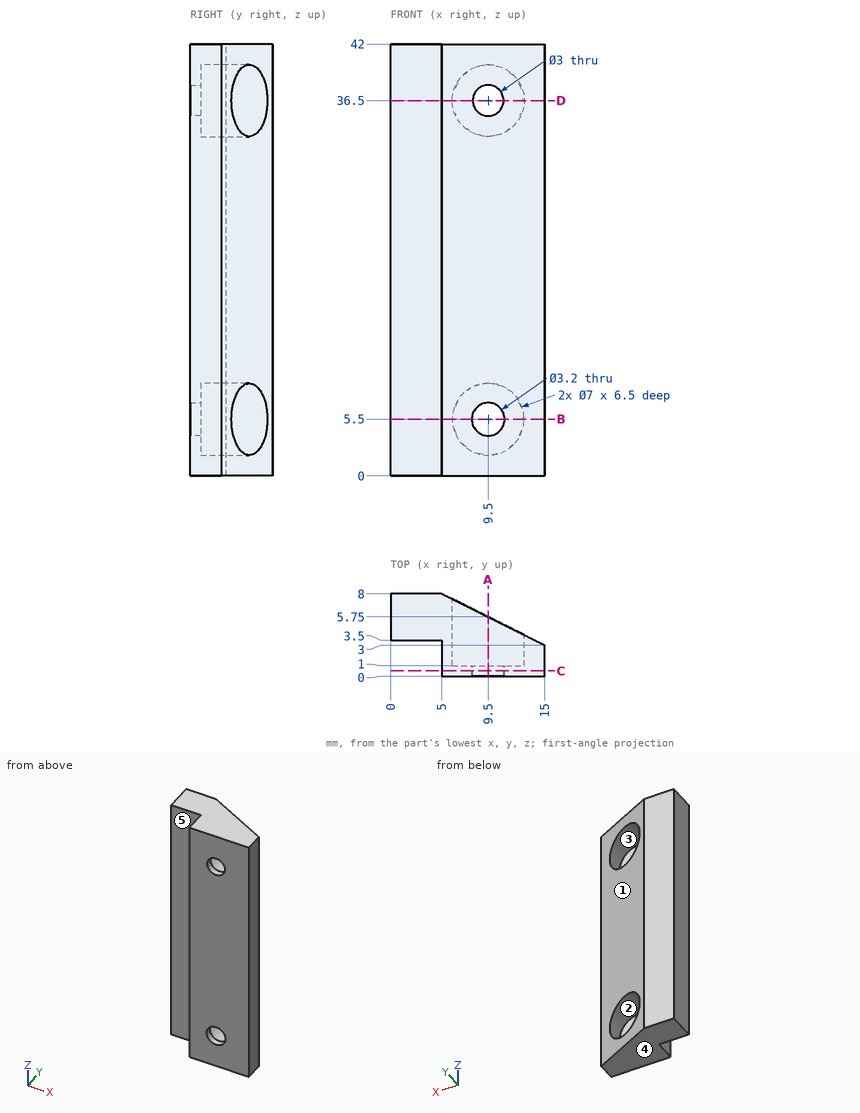
Part print with two shaded views. Sizes in mm from the minimum x, y, z corner. A direction names the side the tool comes from. Round coordinates to 2 decimals unless told otherwise and drop trailing zeros. Write each loop counter-clockwise with the first axis right and the second up, starting at its lowest first coordinate (ties: lowest second). Pieces come first, ordered by that corner, then holes. Notation, with made-up numbers: (21, 83.25) -> (75, 83.25) arc R13 ccw to (75, 100.25) -> close; hole circle Ø11 at (30, 89). An arc over 180 degrees is marked (long way). Use one line per item in the form item = value.
Q1. Band-saw the part on A-A, the plane x = 9.5. Write the cut outline in (y, z), then the cut area to 3 significant figures.
Conclusion:
outline = (0, 0) -> (5.75, 0) -> (5.75, 2) -> (1, 2) -> (1, 3.9) -> (0, 3.9) -> close; (0, 7.1) -> (1, 7.1) -> (1, 9) -> (5.75, 9) -> (5.75, 33) -> (1, 33) -> (1, 35) -> (0, 35) -> close; (0, 38) -> (1, 38) -> (1, 40) -> (5.75, 40) -> (5.75, 42) -> (0, 42) -> close
area = 169 mm²
Q2. Band-saw the part on C-C, the plane y = 0.5. Write the cut outline in (x, z), then the cut area to 3 significant figures.
Conclusion:
outline = (5, 0) -> (15, 0) -> (15, 42) -> (5, 42) -> close; hole circle Ø3.2 at (9.5, 5.5); hole circle Ø3 at (9.5, 36.5)
area = 405 mm²
Q3. Drill centre lines: L1, parallel to Z at x = 9.5, y = 3; L2, parallel to Z at x = 12, y = 3; L3, parallel to Y at x = 7, z = 6. Where is each one in solid material? Low to high.
Conclusion:
L1 = 0 to 2, 9 to 33, 40 to 42
L2 = 0 to 3.05, 7.95 to 34.05, 38.95 to 42
L3 = 0 to 1
Q4. Band-saw the part on B-B, the plane z = 5.5. Write the cut outline in (x, y), then the cut area to 4 significant figures.
Conclusion:
outline = (0, 3.5) -> (5, 3.5) -> (5, 0) -> (7.9, 0) -> (7.9, 1) -> (6, 1) -> (6, 7.5) -> (5, 8) -> (0, 8) -> close; (11.1, 0) -> (15, 0) -> (15, 3) -> (13, 4) -> (13, 1) -> (11.1, 1) -> close
area = 41.05 mm²
Q5. Two-plate mould, pull along Z, no slides. Class the marked faces 3, 4 and 5: released by +Z, released by -Z, zero draft, split by the parting line, or undercut.
Conclusion:
face_3 = undercut
face_4 = released by -Z
face_5 = zero draft
Q6. Drop flat-ended pins along their axis: P1, Ø6, axis at x = 11, z = 26, coming from the +Y side; P2, Ø2, axis at x = 8.5, z = 37.5, coming from the +Y side; P3, Ø5.5, axis at x = 10.5, z = 5, coming from the +Y side. Give the stop position or say it passes through.
Conclusion:
P1 = 6.5
P2 = 1
P3 = 5.07
Q7. Tool access for the marked faces 1 and 2: list every direction of +Z, -Z, +X, -X, +Y, -Y with a clear straight run to the whole face (end or side of a thin tool).
Conclusion:
face_1 = +Z, -Z, +X, +Y
face_2 = +Y
Q8. Band-saw the part on D-D, the plane z = 36.5. Write the cut outline in (x, y).
Conclusion:
outline = (0, 3.5) -> (5, 3.5) -> (5, 0) -> (8, 0) -> (8, 1) -> (6, 1) -> (6, 7.5) -> (5, 8) -> (0, 8) -> close; (11, 0) -> (15, 0) -> (15, 3) -> (13, 4) -> (13, 1) -> (11, 1) -> close
